Read the model definition and answer for the solid it produces. Units are mm, in the model's axes. Face numbers are marked on the shaded views. A direction names the side the tool comes from. Give positions to 0.01 mm unless a question says otherwise; leave off trailing zeros. Write each loop counter-clockwise with the first axis right and the second up, starting at its lowest first coordinate (ties: lowest second). Pieces come first, ordered by that corner, then holes.
```python
from build123d import *

# Parameters (mm, degrees)
BOSS_EXTRUDE1_DEPTH     = 1.3
SKETCH3_W               = 15
SKETCH3_H               = 15
BOSS_EXTRUDE2_DEPTH     = 5.5
SKETCH5_R               = 1.75
CUT_EXTRUDE1_DEPTH      = 14.345785852
BOSS_EXTRUDE3_START     = 1.5
SKETCH8_R               = 1.75
BOSS_EXTRUDE3_DEPTH     = 1.5
SKETCH9_R               = 1.75
BOSS_EXTRUDE4_DEPTH     = 6
CUT_EXTRUDE3_DEPTH      = 4.1
CUT_EXTRUDE4_DEPTH      = 19.712028217
CUT_EXTRUDE4_DEPTH_BACK = 19.712028217
CHAMFER1_SIZE           = 0.5
CHAMFER2_SIZE           = 2
FILLET1_R               = 1
CHAMFER3_SIZE           = 1


with BuildPart() as part:
    # Sketch2 → Boss-Extrude1 (new, symmetric)
    with BuildSketch(Plane(origin=(0, 0, 0), x_dir=(1, 0, 0), z_dir=(0, 1, 0))):
        Polygon((-7.5, 7.5), (7.5, 7.5), (7.5, 3), (4.732050808, 3), (1.267949192, 3), (-0.464101615, 0), (1.267949192, -3), (4.732050808, -3), (7.5, -3), (7.5, -7.5), (-7.5, -7.5), (-7.5, -5.75), (-7.5, 5.75), align=None)
    extrude(amount=BOSS_EXTRUDE1_DEPTH, both=True)

    # Sketch3 → Boss-Extrude2 (add)
    with BuildSketch(Plane(origin=(0, 1.3, 0), x_dir=(1, 0, 0), z_dir=(0, 1, 0))):
        Rectangle(SKETCH3_W, SKETCH3_H)
    extrude(amount=BOSS_EXTRUDE2_DEPTH)

    # Sketch5 → Cut-Extrude1 (cut, through all)
    with BuildSketch(Plane(origin=(0, 6.8, 0), x_dir=(1, 0, 0), z_dir=(0, 1, 0))):
        with Locations(Location((-3.102458521, 3, 0), (0, 0, 270))):
            Circle(SKETCH5_R)
        with Locations(Location((-3.102458521, -3, 0), (0, 0, 270))):
            Circle(SKETCH5_R)
        with Locations(Location((3, 0, 0), (0, 0, 270))):
            Circle(SKETCH5_R)
    extrude(amount=-CUT_EXTRUDE1_DEPTH, mode=Mode.SUBTRACT)

    # Sketch8 → Boss-Extrude3 (add)
    with BuildSketch(Plane(origin=(0, 6.8, 0), x_dir=(1, 0, 0), z_dir=(0, 1, 0)).offset(BOSS_EXTRUDE3_START)):
        Polygon((-7.5, 7.5), (7.5, 7.5), (7.5, 2.75), (7.5, -2.75), (7.5, -7.5), (-7.5, -7.5), (-7.5, -5.75), (-4.690171761, -5.75), (-1.514745281, -5.75), (0.07296796, -3), (-1.514745281, -0.25), (-4.690171761, -0.25), (-7.5, -0.25), (-7.5, 0.25), (-4.690171761, 0.25), (-1.514745281, 0.25), (0.07296796, 3), (-1.514745281, 5.75), (-4.690171761, 5.75), (-7.5, 5.75), align=None)
        with Locations(Location((3, 0, 0), (0, 0, 270))):
            Circle(SKETCH8_R, mode=Mode.SUBTRACT)
    extrude(amount=-BOSS_EXTRUDE3_DEPTH)

    # Sketch9 → Boss-Extrude4 (add)
    with BuildSketch(Plane.XZ.offset(1.3)):
        Polygon((7.5, 3), (7.5, -3), (7.5, -7.5), (-7.5, -7.5), (-7.5, 7.5), (7.5, 7.5), align=None)
        with Locations(Location((-3.102458521, 3, 0), (0, 0, 90))):
            Circle(SKETCH9_R, mode=Mode.SUBTRACT)
        with Locations(Location((-3.102458521, -3, 0), (0, 0, 90))):
            Circle(SKETCH9_R, mode=Mode.SUBTRACT)
    extrude(amount=BOSS_EXTRUDE4_DEPTH)

    # Sketch11 → Cut-Extrude3 (cut)
    with BuildSketch(Plane(origin=(0, 6.8, 0), x_dir=(1, 0, 0), z_dir=(0, 1, 0))):
        Polygon((-7.5, 0.25), (-1.514745281, 0.25), (0.07296796, 3), (-1.514745281, 5.75), (-7.5, 5.75), align=None)
        Polygon((-7.5, -5.75), (-1.514745281, -5.75), (0.07296796, -3), (-1.514745281, -0.25), (-7.5, -0.25), align=None)
    extrude(amount=-CUT_EXTRUDE3_DEPTH, mode=Mode.SUBTRACT)

    # Sketch10 → Cut-Extrude4 (cut, two sides: drawn at the far end of the back side and taken through both)
    with BuildSketch(Plane.XY.offset(7.5).offset(-CUT_EXTRUDE4_DEPTH_BACK)):
        Polygon((0.5, -7.3), (7.5, -1.7), (7.5, -7.3), align=None)
    extrude(amount=CUT_EXTRUDE4_DEPTH + CUT_EXTRUDE4_DEPTH_BACK, mode=Mode.SUBTRACT)

    # Chamfer1
    chamfer1_edges = [part.edges().sort_by_distance(p)[0] for p in [
        (3, 8.3, -1.75),
    ]]
    chamfer(chamfer1_edges, length=CHAMFER1_SIZE)

    # Chamfer2
    chamfer2_edges = [part.edges().sort_by_distance(p)[0] for p in [
        (-7.5, 8.3, 0),
    ]]
    chamfer(chamfer2_edges, length=CHAMFER2_SIZE)

    # Fillet1
    fillet1_edges = [part.edges().sort_by_distance(p)[0] for p in [
        (7.5, 3.3, 7.5),
        (-7.5, 0.5, 7.5),
        (-7.5, 0.5, -7.5),
        (7.5, 3.3, -7.5),
    ]]
    fillet(fillet1_edges, radius=FILLET1_R)

    # Chamfer3
    chamfer3_edges = [part.edges().sort_by_distance(p)[0] for p in [
        (-3, -7.3, 7.5),
        (-7.5, -7.3, 0),
        (-3, -7.3, -7.5),
        (-7.207106781, -7.3, -7.207106781),
        (-7.207106781, -7.3, 7.207106781),
    ]]
    chamfer(chamfer3_edges, length=CHAMFER3_SIZE)


solid = part.part
```
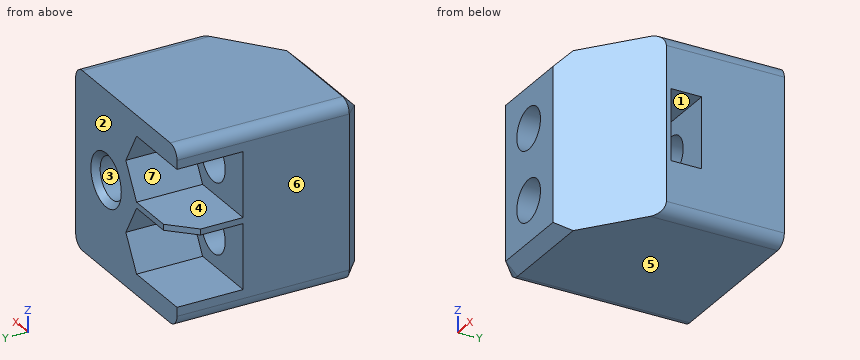
Item 1: Section A-A (x = 6.25) is taken. Write down the section's boundary in (y, z), and give its area (3 significant figures).
Result set:
outline: (-2.7, -7.5) - (8.3, -7.5) - (8.3, 7.5) - (-2.7, 7.5) - close; hole (-1.3, -3) - (1.3, -3) - (1.3, 3) - (-1.3, 3) - close
area: 149 mm2
Item 2: Each of these flat-tipped pins is pushed along its axis until it touches: pin 1 Ø8 at (x, z) = (-4.5, -1.5) entering from +Y; pin 2 Ø3 at (x, z) = (-3.1, 3) entering from -Y; pin 3 Ø4 at (x, z) = (3, 0) entering from +Y; pin 4 Ø4 at (x, z) = (-3.1, -3) entering from +Y. Where does it stop, or does it pass through?
Result set:
pin 1: stops at y = 8.3
pin 2: passes through
pin 3: stops at y = 8.05
pin 4: stops at y = 2.7
Item 3: Section B-B (x = 3) is taken. Write down the section's boundary in (y, z), and give its area (3 significant figures).
Result set:
outline: (-5.3, -7.5) - (8.3, -7.5) - (8.3, -2.25) - (7.8, -1.75) - (1.3, -1.75) - (1.3, -3) - (-1.3, -3) - (-1.3, 3) - (1.3, 3) - (1.3, 1.75) - (7.8, 1.75) - (8.3, 2.25) - (8.3, 7.5) - (-5.3, 7.5) - close
area: 164 mm2
Item 4: Find the intervals of material crossed by line 1 along Z through (x, y) = (-2, 3); line 2 along Z through (x, y) = (6.25, 0.5); line 3 along X through (y, z) = (3.5, 0), in increasing order.
Result set:
line 1: z = -7.5 to -5.75, -0.25 to 0.25, 5.75 to 7.5
line 2: z = -7.5 to -3, 3 to 7.5
line 3: x = -7.5 to 1.25, 4.75 to 7.5
Item 5: Which of the six approach directions +Z, -Z, +X, -X, +Y, -Y give full straight-line access (tool end or side, diameter ignored) to the marked faces 1, 2, 3 and 4?
Result set:
face 1: +X
face 2: +Z, -Z, +X, -X, +Y
face 3: +Y
face 4: -X, +Y
Item 6: Determine the mould class of the marked faces 5, 6 and 7 for opening direction Z: pulls with the +Z half, pulls with the -Z half, needs draft (parallel to the pull), parting line crosses it, or undercut.
Result set:
face 5: pulls with the -Z half
face 6: needs draft
face 7: undercut
Item 7: Section D-D (y = -6) is taken. Write down the section's boundary in (x, z) (3 decimals), and give its area (3 significant figures).
Result set:
outline: (-7.5, -6.5) arc R1 ccw to (-6.5, -7.5) - (2.125, -7.5) - (2.125, 7.5) - (-6.5, 7.5) arc R1 ccw to (-7.5, 6.5) - close; hole circle Ø3.5 at (-3.102, -3); hole circle Ø3.5 at (-3.102, 3)
area: 125 mm2
Item 8: Section C-C (z = 4.5) is taken. Write down the section's boundary in (x, y).
Result set:
outline: (-7.5, -6.3) - (-6.5, -7.3) - (-4, -7.3) - (-4, 2.7) - (-7.5, 2.7) - close; (-2.2, -7.3) - (0.5, -7.3) - (7.5, -1.7) - (7.5, 8.3) - (-0.79, 8.3) - (-0.79, 2.7) - (-2.2, 2.7) - close
